Build history of the part. All positions in model axes, mm. Round coordinates to 2 decimals unless told otherwise and drop trailing zeros. Write each loop counter-clockwise with the first axis right and the second up, starting at its lowest first coordinate (ties: lowest second). Pieces come first, ordered by that corner, then holes.
1) Wall check: probe 1 along Y at (x, z) = (20, 2.9); probe 2 along Y at (x, z) = (-16.5, 1.9); probe 3 along X at (y, z) = (-15.5, 1.6). Give the ranges that are in metal, low to high.
2) Pull direction Y, two halves, no side cores. Call faces 1 (the cylindrical face through (-17.024, -14.868, 2.535)), 2 (the cylindrical face through (-29, 28, 3)), 3 (the flat face through (30, 0, 2)): +Y half, -Y half, draft (parallel to the pull), parting line (faces both ways), or undercut.
3) Saw through at B-B (y = -15.5). Write the cut outline in (x, z).
4) Saw through at D-D (z = 4.25). State how many separate pieces and enclosed holes the cut face has, plus the area to 3 significant figures.
5) Saw through at A-A (x = 0). Write the cut outline in (y, z).
from build123d import *

# Parameters (mm, degrees)
F0_W     = 60
F0_H     = 60
F0_R     = 19
F1_DEPTH = 5
F2_D     = 3.3
F2_DEPTH = 13.8
F2_TIP   = 0.9914200214
F4_D     = 4.4
F4_DEPTH = 13.8
F4_TIP   = 1.3218933619
F5_R     = 5


with BuildPart() as f1:
    # F0 (on Top) → F1 (new body)
    with BuildSketch(Plane.XY):
        Rectangle(F0_W, F0_H)
        Circle(F0_R, mode=Mode.SUBTRACT)
    extrude(amount=F1_DEPTH)

    # F2
    with Locations(Plane(origin=(0, 0, 0), x_dir=(1, 0, 0), z_dir=(0, 0, -1))):
        with Locations((-15.5, -15.5), (15.5, -15.5), (15.5, 15.5), (-15.5, 15.5)):
            Hole(F2_D / 2, depth=F2_DEPTH)
            with Locations((0, 0, -(F2_DEPTH + F2_TIP / 2))):  # 118° drill point
                Cone(0, F2_D / 2, F2_TIP, mode=Mode.SUBTRACT)

    # F4
    with Locations(Plane.XY.offset(5)):
        with Locations((-20, 24.5), (20, 24.5), (20, -25.5), (-20, -25.5)):
            Hole(F4_D / 2, depth=F4_DEPTH)
            with Locations((0, 0, -(F4_DEPTH + F4_TIP / 2))):  # 118° drill point
                Cone(0, F4_D / 2, F4_TIP, mode=Mode.SUBTRACT)

    # F5
    f5_edges = [f1.edges().sort_by_distance(p)[0] for p in [
        (-30, 30, 2.5),
        (30, 30, 2.5),
        (30, -30, 2.5),
        (-30, -30, 2.5),
    ]]
    fillet(f5_edges, radius=F5_R)


solid = f1.part
Evaluation:
1. probe 1: y = -30 to -27.7, -23.3 to 22.3, 26.7 to 30
1. probe 2: y = -30 to -16.81, -14.19 to -9.42, 9.42 to 14.19, 16.81 to 30
1. probe 3: x = -30 to -17.15, -13.85 to -10.99, 10.99 to 13.85, 17.15 to 30
2. face 1: undercut
2. face 2: +Y half
2. face 3: draft
3. outline: (-30, 0) - (-17.15, 0) - (-17.15, 5) - (-30, 5) - close; (-13.85, 0) - (-10.99, 0) - (-10.99, 5) - (-13.85, 5) - close; (10.99, 0) - (13.85, 0) - (13.85, 5) - (10.99, 5) - close; (17.15, 0) - (30, 0) - (30, 5) - (17.15, 5) - close
4. separate pieces: 1
4. enclosed holes: 9
4. area: 2,350 mm2
5. outline: (-30, 0) - (-19, 0) - (-19, 5) - (-30, 5) - close; (19, 0) - (30, 0) - (30, 5) - (19, 5) - close
